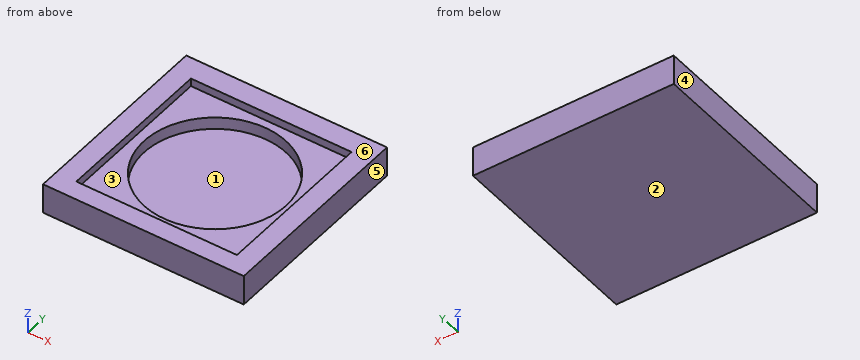
from build123d import *

# Parameters (mm, degrees)
F0_W     = 127
F0_H     = 127
F1_DEPTH = 7.62
F2_W     = 127
F2_H     = 127
F3_DEPTH = 11.43
F4_W     = 101.6
F4_H     = 101.6
F5_DEPTH = 5.08
F6_R     = 44.872379
F7_DEPTH = 7.62


with BuildPart() as f1:
    # F0 (on Top) → F1 (new body)
    with BuildSketch(Plane.XY):
        Rectangle(F0_W, F0_H)
    extrude(amount=F1_DEPTH)

    # F2 (on face) → F3 (join)
    with BuildSketch(Plane.XY.offset(7.62)):
        Rectangle(F2_W, F2_H)
    extrude(amount=F3_DEPTH)

    # F4 (on face) → F5 (cut)
    with BuildSketch(Plane.XY.offset(19.05)):
        with Locations((0, -0.944678)):
            Rectangle(F4_W, F4_H)
    extrude(amount=-F5_DEPTH, mode=Mode.SUBTRACT)

    # F6 (on face) → F7 (cut)
    with BuildSketch(Plane.XY.offset(13.97)):
        Circle(F6_R)
    extrude(amount=-F7_DEPTH, mode=Mode.SUBTRACT)


solid = f1.part
Work out the finished part from the listing and answer in its coordinate system (mm). Face numbers are marked on the shaded views. A direction names the side the tool comes from. Round coordinates to 2 decimals unless told otherwise and drop trailing zeros. Loops run counter-clockwise (first coordinate to the right, second up) from the corner with the lowest first, then second, coordinate; pieces in that order, holes last. Notation, with made-up numbers: M 48.25,35 L 101.25,35 A24 ccw 101.25,56 Z; hole C -38.5,41.25 d1. An arc over 180 degrees is marked long. One line per question, with ' | ' between items. Start each with the question number.
(1) Find the intervals of material crossed by line 1 (Y direction, x = 0, z = 8.5); line 2 (X direction, y = 34, z = 14.5); line 3 (Z direction, x = 22.5, y = -2.5), in increasing order.
(2) A cutting plane is placed at A-A on x = 0. Write down the section's boundary in (y, z), plus the area to 3 significant figures.
(3) A tool of negligible diameter and unlimited length cuts with its end or side. For the marked faces 1 and 2, from which of +Z, -Z, +X, -X, +Y, -Y can it reach the whole face along a straight path? Write none if from no direction.
(4) A cutting plane is placed at B-B on z = 8.75. Write down the section's boundary in (x, y).
(5) For a pull along X with two mould halves and no side action, classify the marked faces 3, 4, 5 and 6 as released by +X, released by -X, zero draft, split by the parting line, or undercut.
(6) A flat-ended cylindrical pin translates along its axis: pin 1 Ø4 at (x, y) = (13.5, -9.5) entering from +Z. Find the tip coordinate at first contact, or state that the pin passes through.
(7) A cutting plane is placed at C-C on y = 0. Write down the section's boundary in (x, z).
Geometry check:
1) line 1: y = -63.5 to -44.87, 44.87 to 63.5 | line 2: x = -63.5 to -50.8, 50.8 to 63.5 | line 3: z = 0 to 6.35
2) outline: M -63.5,0 L 63.5,0 L 63.5,19.05 L 49.86,19.05 L 49.86,13.97 L 44.87,13.97 L 44.87,6.35 L -44.87,6.35 L -44.87,13.97 L -51.74,13.97 L -51.74,19.05 L -63.5,19.05 Z | area: 1,220 mm²
3) face 1: +Z | face 2: -Z, +X, -X, +Y, -Y
4) outline: M -63.5,-63.5 L 63.5,-63.5 L 63.5,63.5 L -63.5,63.5 Z; hole C 0,0 d89.74
5) face 3: undercut | face 4: released by -X | face 5: released by +X | face 6: zero draft
6) pin 1: stops at z = 6.35
7) outline: M -63.5,0 L 63.5,0 L 63.5,19.05 L 50.8,19.05 L 50.8,13.97 L 44.87,13.97 L 44.87,6.35 L -44.87,6.35 L -44.87,13.97 L -50.8,13.97 L -50.8,19.05 L -63.5,19.05 Z
